The model under review builds one solid part; all positions refer to its coordinate system, in mm. Coordinates: 2 decimals unless noted, no trailing zeros. Loops run counter-clockwise (first coordinate to the right, second up) from the corner with the lowest first, then second, coordinate; pieces in that order, holes last. Notation, with made-up numbers: M -13,-11.5 L 7,-11.5 A23 cw 7,10.5 Z; hole C 5,51.5 d10. An arc over 180 degrees is marked long. Use one line per item in the form item = value.
```python
from build123d import *

# Parameters (mm, degrees)
SKETCH1_W              = 132.276038998
SKETCH1_H              = 92.368395504
BOSS_EXTRUDE1_DEPTH    = 25
F_20_0MM_DOWEL_HOLE1_D = 20
F_10_0MM_DOWEL_HOLE1_D = 10


with BuildPart() as part:
    # Sketch1 → Boss-Extrude1 (new body)
    with BuildSketch(Plane.XY):
        Rectangle(SKETCH1_W, SKETCH1_H)
    extrude(amount=BOSS_EXTRUDE1_DEPTH)

    # Ø20.0mm Dowel Hole1 (through all)
    with Locations(Plane.XY.offset(25)):
        with Locations((-30.059973271, 0.936294249)):
            Hole(F_20_0MM_DOWEL_HOLE1_D / 2)

    # Ø10.0mm Dowel Hole1 (through all)
    with Locations(Plane(origin=(0, 46.184197752, 0), x_dir=(1, 0, 0), z_dir=(0, 1, 0))):
        with Locations((34.396494005, -11.366591172)):
            Hole(F_10_0MM_DOWEL_HOLE1_D / 2)


solid = part.part
```
1. The part is to be moulded in two halves that separate along X. For faces 1 (the face through (66.138, -1, 12)), 2 (the face through (-1, 1, 0)), 3 (the face through (39.39, -0.65, 11.15)), say which applies: pulls with the +X half, pulls with the -X half, needs draft (parallel to the pull), parting line crosses it, or undercut.
Response values:
face_1 = pulls with the +X half
face_2 = needs draft
face_3 = undercut
2. Wall thickness on line 1 along Z through (x, y) = (34, 22); line 2 along X through (y, z) = (0.5, 21); line 3 along X through (y, z) = (3, 18): over which ranges is each line inside the solid? List them lowest first. Write a range as from..to.
Response values:
line_1 = 0..6.38, 16.35..25
line_2 = -66.14..-40.05, -20.07..66.14
line_3 = -66.14..-39.84, -20.28..66.14
3. Add section D-D (y = -11.5). State the section outline as (x, z) points.
Response values:
outline = M -66.14,0 L 66.14,0 L 66.14,25 L -66.14,25 Z; hole C 34.4,11.37 d10
4. Add section B-B (y = 8.5). State the section outline as (x, z) points, then the cut area to 3 significant figures.
Response values:
outline = M -66.14,0 L -36.6,0 L -36.6,25 L -66.14,25 Z; M -23.52,0 L 66.14,0 L 66.14,25 L -23.52,25 Z; hole C 34.4,11.37 d10
area = 2,900 mm^2
5. Add section C-C (x = -36.5). State the section outline as (y, z) points, then the cut area to 3 significant figures.
Response values:
outline = M -46.18,0 L -6.71,0 L -6.71,25 L -46.18,25 Z; M 8.59,0 L 46.18,0 L 46.18,25 L 8.59,25 Z
area = 1,930 mm^2
6. Add section A-A (z = 13). State the section outline as (x, y) points.
Response values:
outline = M -66.14,-46.18 L 29.67,-46.18 L 29.67,46.18 L -66.14,46.18 Z; M 39.12,-46.18 L 66.14,-46.18 L 66.14,46.18 L 39.12,46.18 Z; hole C -30.06,0.94 d20
